Part model, mm, in its own coordinate system. Coordinates: 2 decimals unless noted, no trailing zeros. Loops run counter-clockwise (first coordinate to the right, second up) from the corner with the lowest first, then second, coordinate; pieces in that order, holes last. Notation, with made-up numbers: (8.25, 30) - (66.25, 30) arc R18 ccw to (66.25, 36) - close; hole circle Ø4 at (29, 17). An arc over 180 degrees is marked (long way). Use a Markdown table: item, result. Add a question column.
1. Wall check: probe 1 along Y at (x, z) = (2.2, 0); probe 2 along Z at (x, y) = (1.3, 1); probe 3 along Y at (x, z) = (1.9, 0.25). Give the ranges that are in metal, low to high. Write a range as [from, to].
2. Band-saw the part on D-D, the plane z = 3. Give the cut face in (x, y).
3. Band-saw the part on C-C, the plane z = -3.5. Give the cut face in (x, y).
4. Band-saw the part on A-A, the plane x = 1.65. Count the separate pieces of the cut face and the enclosed holes in it, plus the area to 3 significant figures.
5. Pull direction Y, two halves, no side cores. Call faces 1 (the cylindrical face through (1.5, -4.5, -0.1)), 2 (the flat face through (0, 25, -3)), 3 (the cylindrical face through (1.48, -0.97, 1.27)): pulls with the +Y half, pulls with the -Y half, needs draft (parallel to the pull), parting line crosses it, or undercut.
6. Drop a flat-ended pin along its axis: pin 1 (2 mm diameter, centred on y = 25, z = -1.5, fed in from -X). Give the stop position or say it passes through.
from build123d import *

# Parameters (mm, degrees)
SKETCH1_R           = 1.6
SKETCH1_RX          = 17.4
SKETCH1_RY          = 2
BOSS_EXTRUDE1_DEPTH = 3


with BuildPart() as part:
    # Sketch1 → Boss-Extrude1 (new body)
    with BuildSketch(Plane(origin=(0, 0, 0), x_dir=(0, 0, -1), z_dir=(1, 0, 0))):
        with BuildLine():
            Line((-4.5, 0), (-4.5, 50))
            ThreePointArc((-4.5, 50), (0, 54.5), (4.5, 50))
            Line((4.5, 50), (4.5, 0))
            ThreePointArc((4.5, 0), (0, -4.5), (-4.5, 0))
        make_face()
        with Locations((0, 50)):
            Circle(SKETCH1_R, mode=Mode.SUBTRACT)
        Circle(SKETCH1_R, mode=Mode.SUBTRACT)
        with Locations(Location((0, 25), (0, 0, 90))):
            Ellipse(SKETCH1_RX, SKETCH1_RY, mode=Mode.SUBTRACT)
    extrude(amount=BOSS_EXTRUDE1_DEPTH)


solid = part.part
Geometry check:
| question | item | result |
|---|---|---|
| 1 | probe 1 | y = [-4.5, -1.6], [1.6, 7.6], [42.4, 48.4], [51.6, 54.5] |
| 1 | probe 2 | z = [-4.5, -1.25], [1.25, 4.5] |
| 1 | probe 3 | y = [-4.49, -1.58], [1.58, 7.74], [42.26, 48.42], [51.58, 54.49] |
| 2 | outline | (0, -3.35) - (3, -3.35) - (3, 53.35) - (0, 53.35) - close |
| 3 | outline | (0, -2.83) - (3, -2.83) - (3, 52.83) - (0, 52.83) - close |
| 4 | separate pieces | 1 |
| 4 | enclosed holes | 3 |
| 4 | area | 388 mm^2 |
| 5 | face 1 | pulls with the -Y half |
| 5 | face 2 | needs draft |
| 5 | face 3 | undercut |
| 6 | pin 1 | stops at x = 0 |
